Work out the finished part from the listing and answer in its coordinate system (mm). Coordinates: 2 decimals unless noted, no trailing zeros. Order: outer loops, then holes, each group sorted by start corner. A loop starts at its lowest first (then second) coordinate and runs counter-clockwise, first axis right, second up. Notation, with made-up numbers: (3.25, 38) -> (44.25, 38) arc R19 ccw to (44.25, 58) -> close; hole circle Ø4 at (75.5, -17.5). An arc over 180 degrees is marked (long way). Answer as CSV lines item,"result". Start each with the question number.
Item 1: Straight lines are drawn through the part: L1, parallel to X at y = 72, z = -0.5; L2, parallel to Z at x = 0.15, y = -3; L3, parallel to X at y = -66, z = 0.1. For each, find the intervals that lie inside material, in ascending order.
Item 2: Section A-A (y = -37) is taken. Write down the section's boundary in (x, z).
Item 3: Each of these flat-tipped pins is pushed along its axis until it touches: pin 1 Ø0.6 at (x, y) = (0, -33) entering from +Z; pin 2 Ø2 at (x, y) = (1, -30) entering from +Z. Where does it stop, or does it pass through?
```python
from build123d import *

# Parameters (mm, degrees)
SKETCH1_W              = 3
SKETCH1_H              = 170
BASE_FLANGE1_DEPTH     = 1
SKETCHED_START         = -85
SKETCHED_BEND1_DEPTH   = 170
SKETCHED_BEND1_2_DEPTH = 170


# Read off the part's stored shape, not the designer's step: Sketched Bend1
# Sheet-metal steps are written as plain solids
with BuildPart() as part:
    # Sketch1 → Base-Flange1 (new body)
    with BuildSketch(Plane.XY):
        Rectangle(SKETCH1_W, SKETCH1_H)
    extrude(amount=-BASE_FLANGE1_DEPTH)

    # Sketched Bend1 outline → Sketched Bend1 (cut)
    with BuildSketch(Plane(origin=(0, 0, 0), x_dir=(1, 0, 0), z_dir=(0, 1, 0)).offset(SKETCHED_START)):
        with BuildLine():
            ThreePointArc((-1.5, 0.63935721), (-1.000103552, 0.907368803), (-0.440508936, 1))
            Line((-0.440508936, 1), (-1.5, 1))
            Line((-1.5, 1), (-1.5, 0.63935721))
        make_face()
        with BuildLine():
            Line((1.5, 1), (0.258023252, 1))
            ThreePointArc((0.258023252, 1), (0.922591301, 0.867809196), (1.485984888, 0.491361636))
            Line((1.485984888, 0.491361636), (1.5, 0.477346524))
            Line((1.5, 0.477346524), (1.5, 1))
        make_face()
        Polygon((-1.301938308, 0), (-1.5, 0.198061692), (-1.5, 0), align=None)
        Polygon((1.5, 0), (1.5, 0.122473647), (1.377526353, 0), align=None)
    extrude(amount=SKETCHED_BEND1_DEPTH, mode=Mode.SUBTRACT)

    # Sketched Bend1 2 outline → Sketched Bend1 2 (add)
    with BuildSketch(Plane(origin=(0, 0, 0), x_dir=(1, 0, 0), z_dir=(0, 1, 0)).offset(SKETCHED_START)):
        with BuildLine():
            Line((-1.5, 0.198061692), (-1.5, 0.63935721))
            ThreePointArc((-1.5, 0.63935721), (-1.586626572, 0.568081541), (-1.668470572, 0.491361636))
            Line((-1.668470572, 0.491361636), (-1.730885258, 0.42894695))
            Line((-1.730885258, 0.42894695), (-1.5, 0.198061692))
        make_face()
        with BuildLine():
            Line((-0.440508936, 0), (-1.301938308, 0))
            Line((-1.301938308, 0), (-1.023778477, -0.278159831))
            Line((-1.023778477, -0.278159831), (-0.961363791, -0.215745145))
            ThreePointArc((-0.961363791, -0.215745145), (-0.722393552, -0.056070336), (-0.440508936, 0))
        make_face()
        Polygon((1.677436439, 0.299910086), (1.5, 0.477346524), (1.5, 0.122473647), align=None)
        with BuildLine():
            Line((1.377526353, 0), (0.258023252, 0))
            ThreePointArc((0.258023252, 0), (0.539907869, -0.056070336), (0.778878107, -0.215745145))
            Line((0.778878107, -0.215745145), (0.970329658, -0.407196695))
            Line((0.970329658, -0.407196695), (1.377526353, 0))
        make_face()
    extrude(amount=SKETCHED_BEND1_2_DEPTH)


solid = part.part
```
Checked values:
1,L1,"x = -1.66 to 1.48"
1,L2,"z = -1 to 0"
1,L3,"x = -1.2 to -0.81, 0.63 to 1.28"
2,outline,"(-1.73, -0.43) -> (-1.67, -0.49) arc R1.74 ccw to (-0.44, -1) -> (0.26, -1) arc R1.74 ccw to (1.49, -0.49) -> (1.68, -0.3) -> (0.97, 0.41) -> (0.78, 0.22) arc R0.74 cw to (0.26, 0) -> (-0.44, 0) arc R0.74 cw to (-0.96, 0.22) -> (-1.02, 0.28) -> close"
3,pin 1,"stops at z = 0"
3,pin 2,"stops at z = 0.41"
